The model under review builds one solid part; all positions refer to its coordinate system, in mm. Coordinates: 2 decimals unless noted, no trailing zeros. Write each loop counter-clockwise with the first axis right and the second up, starting at its lowest first coordinate (ties: lowest second). Pieces come first, ordered by that corner, then holes.
1) Add section B-B, the plane z = -39. State the section outline as (x, y) points.
2) For P1, Ø2, axis at y = 3.5, z = -44.5, coming from the -X side, flat-tipped, find the tip position at first contact; note if it passes through.
3) For line 1 (Y direction, x = 0, z = -32.5); line 2 (Y direction, x = -4.25, z = -12); line 3 (Y direction, x = -4.75, z = -35), list the stretches that pass through material, from the lowest coordinate up.
4) Add section D-D, the plane y = -5.5. State the section outline as (x, z) points, then the cut area to 3 significant figures.
5) Add section C-C, the plane y = -2.5. State the section outline as (x, z) points, then the cut area to 3 significant figures.
6) Mouldability with a two-part tool opening along Y and no side actions: class faces 1 (the flat face through (3.2, 0.1, 0)), 2 (the cylindrical face through (-3, 0, -27)), 3 (the flat face through (-5.474, 3.219, -27.115)) as released by +Y, released by -Y, zero draft, split by the parting line, or undercut.
7) Add section A-A, the plane x = 0. State the section outline as (y, z) points.
Solid Edge part; units mm, degrees
sketch "Sketch1" plane through (0, 0, 0) normal (0, 0, 1) x (1, 0, 0)
  line L0 (7.3323, 0) -> (3.6662, 6.35)
  line L1 (3.6662, 6.35) -> (-3.6662, 6.35)
  line L2 (-3.6662, 6.35) -> (-7.3323, 0)
  line L3 (-7.3323, 0) -> (-3.6662, -6.35)
  line L4 (-3.6662, -6.35) -> (3.6662, -6.35)
  line L5 (3.6662, -6.35) -> (7.3323, 0)
  circle A0 centre (0, 0) radius 3
extrude "Protrusion1" add sketch "Sketch1" against normal blind 55
properties part number "BumbleB0520"
Geometry results:
1. outline: (-7.33, 0) - (-3.67, -6.35) - (3.67, -6.35) - (7.33, 0) - (3.67, 6.35) - (-3.67, 6.35) - close; hole circle Ø6 at (0, 0)
2. P1: stops at x = -5.89
3. line 1: y = -6.35 to -3, 3 to 6.35
3. line 2: y = -5.34 to 5.34
3. line 3: y = -4.47 to 4.47
4. outline: (-4.16, -55) - (4.16, -55) - (4.16, 0) - (-4.16, 0) - close
4. area: 457 mm2
5. outline: (-5.89, -55) - (-1.66, -55) - (-1.66, 0) - (-5.89, 0) - close; (1.66, -55) - (5.89, -55) - (5.89, 0) - (1.66, 0) - close
5. area: 465 mm2
6. face 1: zero draft
6. face 2: undercut
6. face 3: released by +Y
7. outline: (-6.35, -55) - (-3, -55) - (-3, 0) - (-6.35, 0) - close; (3, -55) - (6.35, -55) - (6.35, 0) - (3, 0) - close
